Could you check a few things on this model? Use its own coordinates, in mm. Face numbers are marked on the shaded views. A direction names the side the tool comes from. Give positions to 0.01 mm unless a question says otherwise; leave off trailing zeros. Loops run counter-clockwise (first coordinate to the right, second up) from the corner with the lowest first, then second, coordinate; pieces in that order, holes last. Notation, with made-up numbers: (-10.75, 75) - (28.25, 75) arc R25 ccw to (28.25, 105) - close; hole circle Ø3 at (12.5, -28.5). An arc over 180 degrees is marked (long way). Answer in a Markdown table with one row per item. Add a question column.
```python
from build123d import *

# Parameters (mm, degrees)
BOSS_EXTRUDE1_DEPTH = 12.7


with BuildPart() as part:
    # Sketch1 → Boss-Extrude1 (new body)
    with BuildSketch(Plane.XY):
        with BuildLine():
            Line((0, 0), (0, 12.7))
            ThreePointArc((0, 12.7), (6.35, 19.05), (12.7, 12.7))
            Line((12.7, 12.7), (12.7, 0))
            Line((12.7, 0), (0, 0))
        make_face()
        with BuildLine():
            Line((1.27, 1.27), (11.43, 1.27))
            Line((11.43, 1.27), (11.43, 12.7))
            ThreePointArc((11.43, 12.7), (6.35, 17.78), (1.27, 12.7))
            Line((1.27, 12.7), (1.27, 1.27))
        make_face(mode=Mode.SUBTRACT)
    extrude(amount=BOSS_EXTRUDE1_DEPTH)


solid = part.part
```
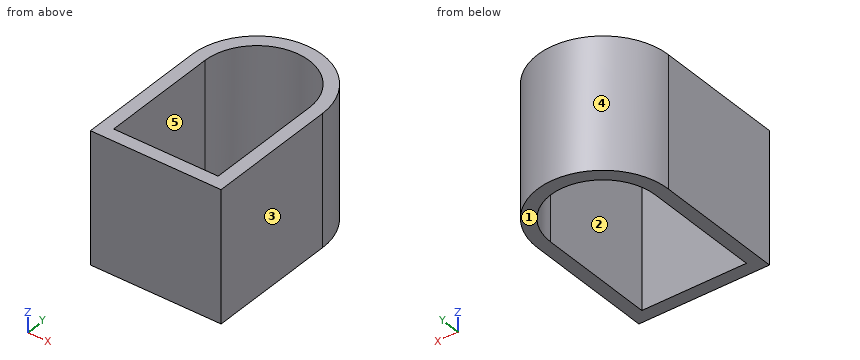
(1) We'd pull the mould along Y, two halves only. Please class the marked faces 3, 4 and 5: pulls with the +Y half, pulls with the -Y half, needs draft (parallel to the pull), parting line crosses it, or undercut.
(2) On a 3-axis mill with a long thin cutter (end or side, diameter ignored), from which of +Z, -Z, +X, -X, +Y, -Y can I reach the whole of each face in a straight line? I mean the marked faces 1 and 2. Say none if no direction works.
(3) Please list where these lines run through material, in increasing order: line 1 (X direction, y = 2.25, z = 4.75); line 2 (Y direction, x = 6.5, z = 3.5); line 3 (Y direction, x = 10.5, z = 2.5).
(4) I want a section at D-D on x = 1. Please give me the cut outline in (y, z).
(5) I want a section at A-A on x = 6.35. Please give me the cut outline in (y, z), then the cut area to 3 significant figures.
(6) I want a section at C-C on y = 11.5. Please give me the cut outline in (x, z).
(7) For pin 1 Ø5 at (x, z) = (8.5, 3.5) entering from +Y, with a flat end and sliding along its axis, tell me the tip position at first contact or that it passes through.
(8) I want a section at B-B on z = 1.25. Please give me the cut outline in (x, y), then the cut area to 3 significant figures.
Reported:
| question | item | result |
|---|---|---|
| 1 | face 3 | needs draft |
| 1 | face 4 | pulls with the +Y half |
| 1 | face 5 | undercut |
| 2 | face 1 | -Z, +X, -X, +Y, -Y |
| 2 | face 2 | +Z, -Z |
| 3 | line 1 | 0 to 1.27, 11.43 to 12.7 |
| 3 | line 2 | 0 to 1.27, 17.78 to 19.05 |
| 3 | line 3 | 0 to 1.27, 15.63 to 17.51 |
| 4 | outline | (0, 0) - (16.12, 0) - (16.12, 12.7) - (0, 12.7) - close |
| 5 | outline | (0, 0) - (1.27, 0) - (1.27, 12.7) - (0, 12.7) - close; (17.78, 0) - (19.05, 0) - (19.05, 12.7) - (17.78, 12.7) - close |
| 5 | area | 32.3 mm² |
| 6 | outline | (0, 0) - (1.27, 0) - (1.27, 12.7) - (0, 12.7) - close; (11.43, 0) - (12.7, 0) - (12.7, 12.7) - (11.43, 12.7) - close |
| 7 | pin 1 | y = 19.05 |
| 8 | outline | (0, 0) - (12.7, 0) - (12.7, 12.7) arc R6.35 ccw to (0, 12.7) - close; hole (1.27, 1.27) - (11.43, 1.27) - (11.43, 12.7) arc R5.08 ccw to (1.27, 12.7) - close |
| 8 | area | 68.0 mm² |
